```python
from build123d import *

# Parameters (mm, degrees)
F1_DEPTH = 48.26
F2_W     = 18.288
F2_H     = 25.4
F3_DEPTH = 10.16
F5_DEPTH = 28.448
F6_R     = 6.35
F6_W     = 51.748991
F6_H     = 25.627352
F7_DEPTH = 38.1


with BuildPart() as f1:
    # F0 (on Top) → F1 (new body)
    with BuildSketch(Plane.XY):
        Polygon((-4.737257, 31.069481), (-33.185257, 31.069481), (-33.185257, 18.369481), (-23.025257, 18.369481), (-23.025257, -17.190519), (-33.185257, -17.190519), (-33.185257, -29.890519), (-4.737257, -29.890519), align=None)
    extrude(amount=F1_DEPTH)

    # F2 (on face) → F3 (cut)
    with BuildSketch(Plane.XY.offset(48.26)):
        with Locations((-13.881257, 0.589481)):
            Rectangle(F2_W, F2_H)
    extrude(amount=-F3_DEPTH, mode=Mode.SUBTRACT)

    # F4 (on Top) → F5 (join)
    with BuildSketch(Plane.XY):
        Polygon((-4.737257, 18.369481), (-4.737257, -17.190519), (55.39888, -17.190519), (86.194743, 0.589481), (55.39888, 18.369481), align=None)
    extrude(amount=F5_DEPTH)

    # F6 (on Front) → F7 (cut, symmetric)
    with BuildSketch(Plane.XZ):
        with Locations((30.314743, 14.224)):
            Circle(F6_R)
        with Locations((92.765238, 30.085676)):
            Rectangle(F6_W, F6_H)
    extrude(amount=F7_DEPTH, both=True, mode=Mode.SUBTRACT)


solid = f1.part
```
Geometry: final body of the model. Coordinates: model frame, mm. A direction names the side the tool comes from. Coordinates: 2 decimals unless noted, no trailing zeros. Order: outer loops, then holes, each group sorted by start corner. A loop starts at its lowest first (then second) coordinate and runs counter-clockwise, first axis right, second up. Notation, with made-up numbers: (17.5, -9.75) -> (41.5, -9.75) arc R9 cw to (41.5, 7.25) -> close; hole circle Ø5 at (-39.75, -4). An arc over 180 degrees is marked (long way). Use CSV: the item, a comma, the result in double quotes.
1) Section A-A on z = 12.5. Output: boundary loops of the cut face in (x, y), then the cut area to 3 significant figures.
Findings:
outline,"(-33.19, -29.89) -> (-4.74, -29.89) -> (-4.74, -17.19) -> (24.2, -17.19) -> (24.2, 18.37) -> (-4.74, 18.37) -> (-4.74, 31.07) -> (-33.19, 31.07) -> (-33.19, 18.37) -> (-23.03, 18.37) -> (-23.03, -17.19) -> (-33.19, -17.19) -> close; (36.43, -17.19) -> (55.4, -17.19) -> (86.19, 0.59) -> (55.4, 18.37) -> (36.43, 18.37) -> close"
area,"3,620 mm^2"
2) Line query: line 1 (X direction, y = 8, z = 34); line 2 (X direction, y = 6.5, z = 25); line 3 (X direction, y = 16.5, z = 10.5). Output: solid intervals per line, ascending.
Findings:
line 1,"x = -23.03 to -4.74"
line 2,"x = -23.03 to 66.89"
line 3,"x = -23.03 to 25.17, 35.46 to 58.64"
3) Pin query (flat end, axial travel): pin 1 Ø5.5 at (x, y) = (-18, -1.5) entering from +Z; pin 2 Ø1.5 at (x, y) = (2, -11.5) entering from -Z; pin 3 Ø11.5 at (x, z) = (30.31, 14.22) entering from -Y; pin 4 Ø5 at (y, z) = (13, 40) entering from -X. Return the tip coordinate at first contact, or that it passes through.
Findings:
pin 1,"stops at z = 38.1"
pin 2,"stops at z = 0"
pin 3,"passes through"
pin 4,"stops at x = -23.03"
4) Section D-D on y = -4. Output: boundary loops of the cut face in (x, z).
Findings:
outline,"(-23.03, 0) -> (78.25, 0) -> (78.25, 17.27) -> (66.89, 17.27) -> (66.89, 28.45) -> (-4.74, 28.45) -> (-4.74, 38.1) -> (-23.03, 38.1) -> close; hole circle Ø12.7 at (30.31, 14.22)"
5) Mould query, pull axis Y, two halves, no side actions, for faces 5 (the flat face through (26, 18.369, 20)), 6 (the flat face through (-14, -12.111, 43)), 7 (the flat face through (-28, -17.191, 24)), 8 (the flat face through (66.891, 0, 23)). Classes: +Y half, -Y half, draft (parallel to the pull), parting line (faces both ways), or undercut.
Findings:
face 5,"+Y half"
face 6,"undercut"
face 7,"undercut"
face 8,"draft"
6) Section B-B on x = -15.5. Output: boundary loops of the cut face in (y, z), then the cut area to 3 significant figures.
Findings:
outline,"(-29.89, 0) -> (31.07, 0) -> (31.07, 48.26) -> (13.29, 48.26) -> (13.29, 38.1) -> (-12.11, 38.1) -> (-12.11, 48.26) -> (-29.89, 48.26) -> close"
area,"2,680 mm^2"
7) Access query for faces 1 (the flat face through (-23.025, 1, 18)), 2 (the flat face through (-14, 13.289, 43)), 3 (the flat face through (25, -17.191, 8)), 4 (the flat face through (31, 1, 28.448)). Directions: +Z, -Z, +X, -X, +Y, -Y. A direction counts if a zero-diameter tool reaches every point of the face in a straight line with its end or side. Return the directions, or none.
Findings:
face 1,"+Z, -Z, -X"
face 2,"+Z, +X, -X"
face 3,"+Z, -Z, +X, -Y"
face 4,"+Z, +X, +Y, -Y"
8) Section C-C on z = 32. Output: boundary loops of the cut face in (x, y), then the cut area to 3 significant figures.
Findings:
outline,"(-33.19, -29.89) -> (-4.74, -29.89) -> (-4.74, 31.07) -> (-33.19, 31.07) -> (-33.19, 18.37) -> (-23.03, 18.37) -> (-23.03, -17.19) -> (-33.19, -17.19) -> close"
area,"1,370 mm^2"
